```python
from build123d import *

# Parameters (mm, degrees)
PAD_DEPTH    = 90
SKETCH001_W  = 24
SKETCH001_H  = 7
POCKET_DEPTH = 2
SKETCH002_R  = 25
PAD001_DEPTH = 13
FILLET_R     = 1
FILLET001_R  = 2
FILLET002_R  = 5
SKETCH003_R  = 5
PAD002_DEPTH = 20
FILLET003_R  = 2


with BuildPart() as part:
    # Sketch → Pad (new body)
    with BuildSketch(Plane.XZ):
        Polygon((-32.625, 33), (32.625, 33), (33.825, 0), (-33.825, 0), align=None)
    extrude(amount=-PAD_DEPTH)

    # Sketch001 (on Face5 of Pad) → Pocket (cut)
    with BuildSketch(Plane.XZ):
        with Locations((0, 21.5)):
            Rectangle(SKETCH001_W, SKETCH001_H)
    extrude(amount=-POCKET_DEPTH, mode=Mode.SUBTRACT)

    # Sketch002 (on Face1 of Pocket) → Pad001 (join)
    with BuildSketch(Plane(origin=(0, 0, 33), x_dir=(-1, 0, 0), z_dir=(0, 0, 1))):
        with Locations((0, -29)):
            Circle(SKETCH002_R)
    extrude(amount=PAD001_DEPTH)

    # Fillet
    fillet_edges = [part.edges().sort_by_distance(p)[0] for p in [
        (25, 29, 46),
    ]]
    fillet(fillet_edges, radius=FILLET_R)

    # Fillet001
    fillet001_edges = [part.edges().sort_by_distance(p)[0] for p in [
        (25, 29, 33),
    ]]
    fillet(fillet001_edges, radius=FILLET001_R)

    # Fillet002
    fillet002_edges = [part.edges().sort_by_distance(p)[0] for p in [
        (33.225, 0, 16.5),
        (33.225, 90, 16.5),
        (-33.225, 0, 16.5),
        (-33.225, 90, 16.5),
    ]]
    fillet(fillet002_edges, radius=FILLET002_R)

    # Sketch003 (on Face6 of Fillet002) → Pad002 (join)
    with BuildSketch(Plane(origin=(0, 90, 0), x_dir=(1, 0, 0), z_dir=(0, 1, 0))):
        with Locations((0, -20.5)):
            Circle(SKETCH003_R)
    extrude(amount=PAD002_DEPTH)

    # Fillet003
    fillet003_edges = [part.edges().sort_by_distance(p)[0] for p in [
        (-5, 90, 20.5),
    ]]
    fillet(fillet003_edges, radius=FILLET003_R)


solid = part.part
```
Model file for the job. Use its own axes, mm. A direction names the side the tool comes from. Coordinates: 2 decimals unless noted, no trailing zeros. Loops run counter-clockwise (first coordinate to the right, second up) from the corner with the lowest first, then second, coordinate; pieces in that order, holes last. Notation, with made-up numbers: (38.25, 37) - (61.25, 37) arc R23 cw to (61.25, 61) - close; hole circle Ø11 at (66.25, -26). An arc over 180 degrees is marked (long way). Answer as a JSON object with one key per item and string values. Group by question number.
(1) Cut at C-C (z = 40). Give the cut face in (x, y), then the cut area to 3 significant figures.
(2) Cut at B-B (x = 0). Give the cut face in (y, z).
(3) Two-plate mould, pull along X, no slides. Class faces 1 (the face through (0, 44, 0)), 2 (the face through (0, 2, 22)), 3 (the face through (33.217, 44.44, 16.731)): released by +X, released by -X, zero draft, split by the parting line, or undercut.
(4) Cut at A-A (y = 29). Give the cut face in (x, z) (3 decimals).
(5) Tool access for faces 4 (the face through (5.42, 53.406, 39.93)), 5 (the face through (-1.08, 100.87, 25.38)), 6 (the face through (0, 110, 20)): list every direction of +Z, -Z, +X, -X, +Y, -Y with a clear straight run to the whole face (end or side of a thin tool).
(6) Probe line 1 along Y through (x, z) = (-10.5, 6); line 2 along Z through (x, y) = (-28.5, 13); line 3 along X through (y, z) = (37, 44). List the from-to ranges inside material, lowest first.
(7) Flat gauge pins, fed straight in: pin 1 (1.5 mm diameter, centred on y = 43.5, z = 36.5, fed in from +X); pin 2 (2 mm diameter, centred on y = 1, z = 21.5, fed in from +X); pin 3 (12 mm diameter, centred on x = -6.5, z = 31.5, fed in from +Y). Where does each tip first touch, or does it go through?
(8) Cut at D-D (y = 101). Give the cut face in (x, z).
Geometry says:
{
 "1": {"outline": "circle Ø50 at (0, 29)", "area": "1,960 mm^2"},
 "2": {"outline": "(0, 0) - (90, 0) - (90, 13.5) arc R2 cw to (92, 15.5) - (110, 15.5) - (110, 25.5) - (92, 25.5) arc R2 cw to (90, 27.5) - (90, 33) - (56, 33) arc R2 cw to (54, 35) - (54, 45) arc R1 ccw to (53, 46) - (5, 46) arc R1 ccw to (4, 45) - (4, 35) arc R2 cw to (2, 33) - (0, 33) - (0, 25) - (2, 25) - (2, 18) - (0, 18) - close"},
 "3": {"face 1": "zero draft", "face 2": "undercut", "face 3": "released by +X"},
 "4": {"outline": "(-33.825, 0) - (33.825, 0) - (32.625, 33) - (27, 33) arc R2 cw to (25, 35) - (25, 45) arc R1 ccw to (24, 46) - (-24, 46) arc R1 ccw to (-25, 45) - (-25, 35) arc R2 cw to (-27, 33) - (-32.625, 33) - close"},
 "5": {"face 4": "+Z", "face 5": "+Y", "face 6": "+Z, -Z, +X, -X, +Y"},
 "6": {"line 1": "y = 0 to 90", "line 2": "z = 0 to 33", "line 3": "x = -23.69 to 23.69"},
 "7": {"pin 1": "stops at x = 20.88", "pin 2": "stops at x = 32.04", "pin 3": "stops at y = 90.01"},
 "8": {"outline": "circle Ø10 at (0, 20.5)"}
}
